For this review, use the dimensioned drawing (mm, ordinates from the lowest corner) and the shaded views. A direction names the side the tool comes from. Give positions to 0.01 mm unless a question says otherwise; leave off trailing zeros. Loops run counter-clockwise (first coordinate to the right, second up) from the corner with the lowest first, then second, coordinate; pieces in that order, holes last. Notation, with made-up numbers: (-39.75, 16) -> (-1.75, 16) arc R9 ccw to (-1.75, 26) -> close; hole circle Ø2 at (58.25, 4). An arc over 180 degrees is marked (long way). Write each question's results on one line, items separated by ' | '. Start each with the question number.
Q1. We need section A-A (z = 2). Write out the cut boundary in (x, y).
Q2. Machinability: for the marked faces 5, 6, 7 and 8, which of the approach directions +Z, -Z, +X, -X, +Y, -Y give a long, thin tool a straight path to every point of the face, cutting with its end or side? Answer none if there is none.
Q3. Mouldability with a two-part tool opening along Y and no side actions: class the marked faces 1, 2, 3 and 4 as released by +Y, released by -Y, zero draft, split by the parting line, or undercut.
Q4. We need section C-C (x = 9.5). Write out the cut boundary in (y, z).
Q5. We need section D-D (z = 15.8). Write out the cut boundary in (x, y) (3 decimals).
Q6. We need section B-B (y = 28.5). Write out the cut boundary in (x, z) (1 decimal).
Q7. Wall thickness on L1, parallel to Y at x = 1.75, z = 5.25; L2, parallel to Z at x = 9.75, y = 54; L3, parallel to X at y = 35, z = 11.75 (3 decimals): over which ranges is each line inside the solid? List them lowest first. Write a range as [from, to].
Q8. Insertion check: pin 1 Ø5.5 at (y, z) = (26.5, 15) entering from +X (3 decimals); pin 2 Ø4 at (y, z) = (52.5, 6) entering from -X; pin 3 Ø6 at (x, y) = (11.5, 42.5) entering from -Z; pin 4 Ø1 at (x, y) = (13, 50.5) entering from +Z. Each pin has a flat end and moves straight along its axis. Give the tip position at first contact, or say it passes through.
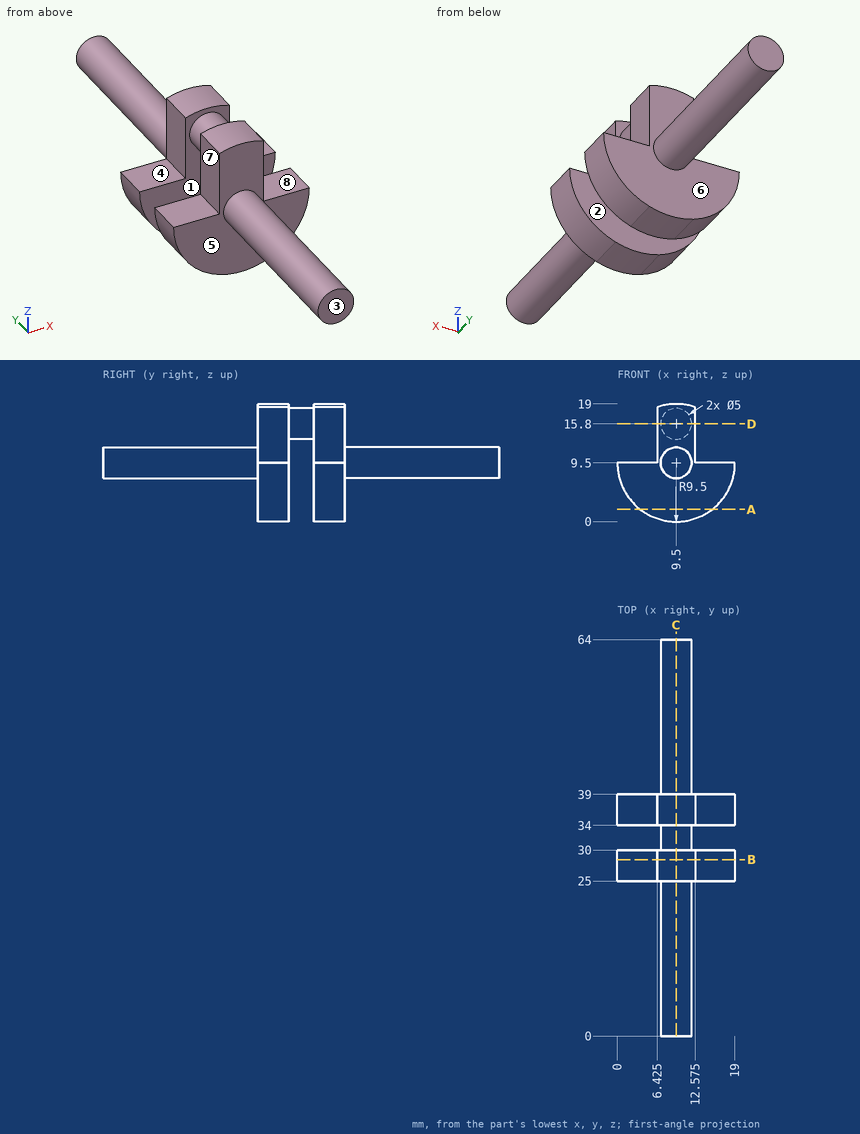
Output:
1) outline: (3.67, 25) -> (15.33, 25) -> (15.33, 30) -> (3.67, 30) -> close; (3.67, 34) -> (15.33, 34) -> (15.33, 39) -> (3.67, 39) -> close
2) face 5: -Y | face 6: +Y | face 7: +Z, -X, +Y, -Y | face 8: +Z, +X, +Y, -Y
3) face 1: undercut | face 2: undercut | face 3: released by -Y | face 4: zero draft
4) outline: (0, 7) -> (25, 7) -> (25, 0) -> (30, 0) -> (30, 13.3) -> (34, 13.3) -> (34, 0) -> (39, 0) -> (39, 7) -> (64, 7) -> (64, 12) -> (39, 12) -> (39, 19) -> (34, 19) -> (34, 18.3) -> (30, 18.3) -> (30, 19) -> (25, 19) -> (25, 12) -> (0, 12) -> close
5) outline: (6.425, 25) -> (12.575, 25) -> (12.575, 30) -> (12, 30) -> (12, 34) -> (12.575, 34) -> (12.575, 39) -> (6.425, 39) -> (6.425, 34) -> (7, 34) -> (7, 30) -> (6.425, 30) -> close
6) outline: (0, 9.5) arc R9.5 ccw to (19, 9.5) -> (12.6, 9.5) -> (12.6, 18.5) arc R9.5 ccw to (6.4, 18.5) -> (6.4, 9.5) -> close
7) L1: [25, 30], [34, 39] | L2: [7.01, 11.99] | L3: [6.425, 12.575]
8) pin 1: x = 12.575 | pin 2: x = 7.5 | pin 3: z = 7 | pin 4: through
